Autodesk Inventor part; units mm, degrees
ref_plane "YZ Plane" through (0, 0, 0) normal (1, 0, 0) x (0, 1, 0)
ref_plane "XZ Plane" through (0, 0, 0) normal (0, 1, 0) x (-1, 0, 0)
ref_plane "XY Plane" through (0, 0, 0) normal (0, 0, 1) x (1, 0, 0)
sketch "Sketch1" plane through (0, 0, 0) normal (0, 0, 1) x (1, 0, 0)
  circle A0 centre (0, 0) radius 11
  circle A1 centre (0, 0) radius 9.38
  dimension "d0" = 22
  dimension "d2" = 1.62
extrude "Extrusion1" add sketch "Sketch1" along normal blind 759
sketch "Sketch6" plane through (0, 0, 759) normal (0, 0, 1) x (1, 0, 0)
  circle A0 centre (0, 0) radius 9.38
  circle A1 centre (0, 0) radius 11
  line L0 (-3.2787, 10.5) -> (3.2787, 10.5)
  dimension "d18" = 10.5
extrude "Extrusion3" cut sketch "Sketch6" against normal through all contours L0 A1 picked at (-0.3693, 10.648)
sketch "Sketch7" plane through (-3.2787, 10.5, 759) normal (0, 1, 0) x (1, 0, 0)
  circle A0 centre (3.2787, 857) radius 1.27
  line L0 (0, 0) -> (0, 759)
  circle A1 centre (3.2787, 707) radius 1.27
  circle A2 centre (3.2787, 557) radius 1.27
  point P0 (3.2787, 759)
  dimension "d34" = 150
  dimension "d47" = 52
  dimension "d48" = 150
hole "Hole3" at (0, 10.5, -98) at (0, 10.5, 52) at (0, 10.5, 202) direction (0, -1, 0) diameter 3.175 end through all
properties part number "2f2barm" material "PVC-Piping"
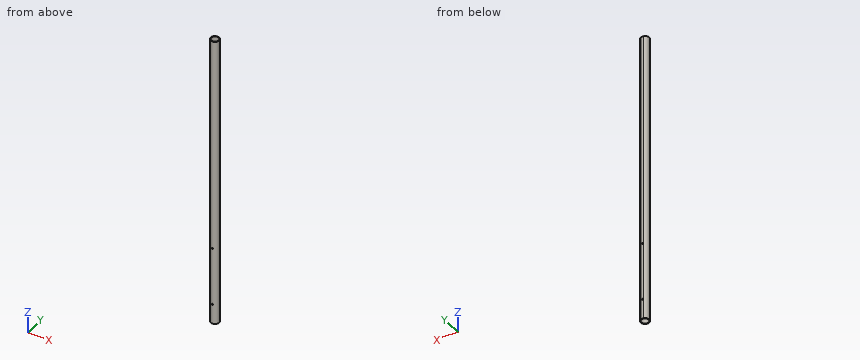
Could you check a few things on this model? Use its own coordinates, in mm. Round coordinates to 2 decimals unless told otherwise and drop trailing zeros. Order: outer loops, then holes, each group sorted by start corner. A loop starts at its lowest first (then second) coordinate and runs counter-clockwise, first axis right, second up.
(1) Imagine slicing it at A-A (y = 0). Write out the boundary of the cut face in (x, z), plus the area to 3 significant figures.
Response values:
outline: (-11, 0) - (-9.38, 0) - (-9.38, 759) - (-11, 759) - close; (9.38, 0) - (11, 0) - (11, 759) - (9.38, 759) - close
area: 2,460 mm2
(2) Imagine slicing it at B-B (z = 485). Write out the boundary of the cut face in (x, y).
Response values:
outline: (-3.28, 10.5) arc R11 ccw (long way) to (3.28, 10.5) - close; hole circle Ø18.76 at (0, 0)
(3) Please list where these lines run through material, in increasing order: line 1 along Z through (x, y) = (0, 9.95); line 2 along Y through (x, z) = (1.25, 57); line 3 along Y through (x, z) = (0.25, 694.5).
Response values:
line 1: z = 0 to 50.41, 53.59 to 200.41, 203.59 to 759
line 2: y = -10.93 to -9.3, 9.3 to 10.5
line 3: y = -11 to -9.38, 9.38 to 10.5
(4) I'm going to push flat-ended pins straight in: pin 1 (10 mm diameter, centred on x = -7, z = 655, fed in from -Y); pin 2 (4 mm diameter, centred on y = -4.5, z = 451, fed in from +X); pin 3 (1 mm diameter, centred on y = -7.5, z = 151, fed in from -X); pin 4 (5 mm diameter, centred on x = -1, y = 4.5, fed in from -Z). Where does each tip first touch, or does it pass through?
Response values:
pin 1: stops at y = -10.82
pin 2: stops at x = 10.71
pin 3: stops at x = -8.49
pin 4: passes through
